```python
from build123d import *

# Parameters (mm, degrees)
SKETCH1_R               = 1.75
SKETCH1_W               = 5
SKETCH1_H               = 20
SKETCH1_R_2             = 13
BOSS_EXTRUDE1_DEPTH     = 3
SKETCH3_R               = 7.5
SKETCH3_R_2             = 4.75
BOSS_EXTRUDE2_DEPTH     = 8
BOSS_EXTRUDE4_DEPTH     = 6
CUT_EXTRUDE3_DEPTH      = 21
CUT_EXTRUDE3_DEPTH_BACK = 10
SKETCH1_5_R             = 1.75
CUT_EXTRUDE4_REACH      = 163.251
SKETCH10_R              = 6
CUT_EXTRUDE5_REACH      = 163.251
SKETCH11_R              = 6


with BuildPart() as part:
    # Sketch1 → Boss-Extrude1 (new body)
    with BuildSketch(Plane.XY):
        with BuildLine():
            Line((45.254833996, 60.811183182), (24.04163056, 39.597979746))
            Line((24.04163056, 39.597979746), (19.192388155, 34.748737342))
            ThreePointArc((19.192388155, 34.748737342), (15.948154667, 32.581009828), (12.121320344, 31.819805153))
            Line((12.121320344, 31.819805153), (-12.121320344, 31.819805153))
            ThreePointArc((-12.121320344, 31.819805153), (-15.948154667, 32.581009828), (-19.192388155, 34.748737342))
            Line((-19.192388155, 34.748737342), (-24.04163056, 39.597979746))
            Line((-24.04163056, 39.597979746), (-45.254833996, 60.811183182))
            Line((-45.254833996, 60.811183182), (-60.811183182, 45.254833996))
            Line((-60.811183182, 45.254833996), (-39.597979746, 24.04163056))
            Line((-39.597979746, 24.04163056), (-34.748737342, 19.192388155))
            ThreePointArc((-34.748737342, 19.192388155), (-32.581009828, 15.948154667), (-31.819805153, 12.121320344))
            Line((-31.819805153, 12.121320344), (-31.819805153, -12.121320344))
            ThreePointArc((-31.819805153, -12.121320344), (-32.581009828, -15.948154667), (-34.748737342, -19.192388155))
            Line((-34.748737342, -19.192388155), (-39.597979746, -24.04163056))
            Line((-39.597979746, -24.04163056), (-60.811183182, -45.254833996))
            Line((-60.811183182, -45.254833996), (-45.254833996, -60.811183182))
            Line((-45.254833996, -60.811183182), (-24.04163056, -39.597979746))
            Line((-24.04163056, -39.597979746), (-19.192388155, -34.748737342))
            ThreePointArc((-19.192388155, -34.748737342), (-15.948154667, -32.581009828), (-12.121320344, -31.819805153))
            Line((-12.121320344, -31.819805153), (12.121320344, -31.819805153))
            ThreePointArc((12.121320344, -31.819805153), (15.948154667, -32.581009828), (19.192388155, -34.748737342))
            Line((19.192388155, -34.748737342), (24.04163056, -39.597979746))
            Line((24.04163056, -39.597979746), (45.254833996, -60.811183182))
            Line((45.254833996, -60.811183182), (60.811183182, -45.254833996))
            Line((60.811183182, -45.254833996), (39.597979746, -24.04163056))
            Line((39.597979746, -24.04163056), (34.748737342, -19.192388155))
            ThreePointArc((34.748737342, -19.192388155), (32.581009828, -15.948154667), (31.819805153, -12.121320344))
            Line((31.819805153, -12.121320344), (31.819805153, 12.121320344))
            ThreePointArc((31.819805153, 12.121320344), (32.581009828, 15.948154667), (34.748737342, 19.192388155))
            Line((34.748737342, 19.192388155), (39.597979746, 24.04163056))
            Line((39.597979746, 24.04163056), (60.811183182, 45.254833996))
            Line((60.811183182, 45.254833996), (45.254833996, 60.811183182))
        make_face()
        with Locations((-40.305086528, -51.618795027)):
            Circle(SKETCH1_R, mode=Mode.SUBTRACT)
        with Locations((-51.618795027, -40.305086528)):
            Circle(SKETCH1_R, mode=Mode.SUBTRACT)
        with Locations((-26.162950904, -37.476659403)):
            Circle(SKETCH1_R, mode=Mode.SUBTRACT)
        with Locations((-37.476659403, -26.162950904)):
            Circle(SKETCH1_R, mode=Mode.SUBTRACT)
        with Locations((-15.25, -15.25)):
            Circle(SKETCH1_R, mode=Mode.SUBTRACT)
        with Locations((26.162950904, -37.476659403)):
            Circle(SKETCH1_R, mode=Mode.SUBTRACT)
        with Locations((40.305086528, -51.618795027)):
            Circle(SKETCH1_R, mode=Mode.SUBTRACT)
        with Locations((51.618795027, -40.305086528)):
            Circle(SKETCH1_R, mode=Mode.SUBTRACT)
        with Locations((15.25, -15.25)):
            Circle(SKETCH1_R, mode=Mode.SUBTRACT)
        with Locations((37.476659403, -26.162950904)):
            Circle(SKETCH1_R, mode=Mode.SUBTRACT)
        with Locations((-37.476659403, 26.162950904)):
            Circle(SKETCH1_R, mode=Mode.SUBTRACT)
        with Locations((-26.162950904, 0)):
            Rectangle(SKETCH1_W, SKETCH1_H, mode=Mode.SUBTRACT)
        with Locations((-15.25, 15.25)):
            Circle(SKETCH1_R, mode=Mode.SUBTRACT)
        with Locations((-51.618795027, 40.305086528)):
            Circle(SKETCH1_R, mode=Mode.SUBTRACT)
        with Locations((-40.305086528, 51.618795027)):
            Circle(SKETCH1_R, mode=Mode.SUBTRACT)
        with Locations((-26.162950904, 37.476659403)):
            Circle(SKETCH1_R, mode=Mode.SUBTRACT)
        Circle(SKETCH1_R_2, mode=Mode.SUBTRACT)
        with Locations((26.162950904, 0)):
            Rectangle(SKETCH1_W, SKETCH1_H, mode=Mode.SUBTRACT)
        with Locations((15.25, 15.25)):
            Circle(SKETCH1_R, mode=Mode.SUBTRACT)
        with Locations((37.476659403, 26.162950904)):
            Circle(SKETCH1_R, mode=Mode.SUBTRACT)
        with Locations((26.162950904, 37.476659403)):
            Circle(SKETCH1_R, mode=Mode.SUBTRACT)
        with Locations((51.618795027, 40.305086528)):
            Circle(SKETCH1_R, mode=Mode.SUBTRACT)
        with Locations((40.305086528, 51.618795027)):
            Circle(SKETCH1_R, mode=Mode.SUBTRACT)
    extrude(amount=BOSS_EXTRUDE1_DEPTH)

    # Sketch3 → Boss-Extrude2 (add)
    # profile 1 of 4: a face of its own
    with BuildSketch(Plane.XY):
        with Locations((-40.001785669, 40.001785669)):
            Circle(SKETCH3_R)
        with Locations((-40.001785669, 40.001785669)):
            Circle(SKETCH3_R_2, mode=Mode.SUBTRACT)
    # profile 2 of 4: a face of its own
    with BuildSketch(Plane.XY):
        with Locations(Location((-40.001785669, -40.001785669, 0), (0, 0, 180))):
            Circle(SKETCH3_R)
        with Locations((-40.001785669, -40.001785669)):
            Circle(SKETCH3_R_2, mode=Mode.SUBTRACT)
    # profile 3 of 4: a face of its own
    with BuildSketch(Plane.XY):
        with Locations((40.001785669, -40.001785669)):
            Circle(SKETCH3_R)
        with Locations((40.001785669, -40.001785669)):
            Circle(SKETCH3_R_2, mode=Mode.SUBTRACT)
    # profile 4 of 4: a face of its own
    with BuildSketch(Plane.XY):
        with Locations(Location((40.001785669, 40.001785669, 0), (0, 0, 180))):
            Circle(SKETCH3_R)
        with Locations((40.001785669, 40.001785669)):
            Circle(SKETCH3_R_2, mode=Mode.SUBTRACT)
    extrude(amount=-BOSS_EXTRUDE2_DEPTH)

    # Sketch7 → Boss-Extrude4 (add)
    with BuildSketch(Plane.XY.offset(3)):
        Polygon((-34.748737342, 19.192388155), (-19.192388155, 34.748737342), (-45.254833996, 60.811183182), (-60.811183182, 45.254833996), align=None)
        Polygon((-60.811183182, -45.254833996), (-34.748737342, -19.192388155), (-19.192388155, -34.748737342), (-45.254833996, -60.811183182), align=None)
        Polygon((34.748737342, -19.192388155), (19.192388155, -34.748737342), (45.254833996, -60.811183182), (60.811183182, -45.254833996), align=None)
        Polygon((60.811183182, 45.254833996), (34.748737342, 19.192388155), (19.192388155, 34.748737342), (45.254833996, 60.811183182), align=None)
    extrude(amount=BOSS_EXTRUDE4_DEPTH)

    # Sketch1<5> → Cut-Extrude3 (cut, two sides: drawn at the far end of the back side and taken through both)
    with BuildSketch(Plane.XY.offset(-CUT_EXTRUDE3_DEPTH_BACK)):
        with Locations(Location((-37.476659403, -26.162950904, 0), (0, 0, 180))):
            Circle(SKETCH1_5_R)
        with Locations(Location((-26.162950904, -37.476659403, 0), (0, 0, 180))):
            Circle(SKETCH1_5_R)
        with Locations(Location((-40.305086528, -51.618795027, 0), (0, 0, 180))):
            Circle(SKETCH1_5_R)
        with Locations(Location((-51.618795027, -40.305086528, 0), (0, 0, 180))):
            Circle(SKETCH1_5_R)
        with Locations(Location((26.162950904, 37.476659403, 0), (0, 0, 180))):
            Circle(SKETCH1_5_R)
        with Locations(Location((37.476659403, 26.162950904, 0), (0, 0, 180))):
            Circle(SKETCH1_5_R)
        with Locations(Location((51.618795027, 40.305086528, 0), (0, 0, 180))):
            Circle(SKETCH1_5_R)
        with Locations(Location((40.305086528, 51.618795027, 0), (0, 0, 180))):
            Circle(SKETCH1_5_R)
        with Locations((40.305086528, -51.618795027)):
            Circle(SKETCH1_5_R)
        with Locations((51.618795027, -40.305086528)):
            Circle(SKETCH1_5_R)
        with Locations((37.476659403, -26.162950904)):
            Circle(SKETCH1_5_R)
        with Locations((26.162950904, -37.476659403)):
            Circle(SKETCH1_5_R)
        with Locations((-51.618795027, 40.305086528)):
            Circle(SKETCH1_5_R)
        with Locations((-40.305086528, 51.618795027)):
            Circle(SKETCH1_5_R)
        with Locations((-26.162950904, 37.476659403)):
            Circle(SKETCH1_5_R)
        with Locations((-37.476659403, 26.162950904)):
            Circle(SKETCH1_5_R)
    extrude(amount=CUT_EXTRUDE3_DEPTH + CUT_EXTRUDE3_DEPTH_BACK, mode=Mode.SUBTRACT)

    # Cut-Extrude4: up to this face of the body (flat: up to its plane)
    cut_extrude4_end = Plane(part.part.faces().sort_by_distance((53.033008589, -53.033008589, 4.5))[0])
    # Sketch10 → Cut-Extrude4 (cut, up to the picked face)
    with BuildSketch(Plane(origin=(-53.033008589, 53.033008589, 0), x_dir=(0, 0, 1), z_dir=(-0.7071067811865477, 0.7071067811865474, 0)), mode=Mode.PRIVATE) as cut_extrude4_sk1:
        with Locations((11.5, 0)):
            Circle(SKETCH10_R)
    cut_extrude4_tool1 = split(extrude(cut_extrude4_sk1.sketch, amount=-CUT_EXTRUDE4_REACH, mode=Mode.PRIVATE), bisect_by=cut_extrude4_end, keep=Keep.BOTH, mode=Mode.PRIVATE)
    add(cut_extrude4_tool1.solids().sort_by(Axis((-53.033009, 53.033009, 11.5), (0.7071067811865477, -0.7071067811865474, 0)))[0], mode=Mode.SUBTRACT)

    # Cut-Extrude5: up to this face of the body (flat: up to its plane)
    cut_extrude5_end = Plane(part.part.faces().sort_by_distance((-53.033008589, -53.033008589, 4.5))[0])
    # Sketch11 → Cut-Extrude5 (cut, up to the picked face)
    with BuildSketch(Plane(origin=(53.033008589, 53.033008589, 0), x_dir=(0.7071067811865552, -0.7071067811865398, 0), z_dir=(0.7071067811865398, 0.7071067811865552, 0)), mode=Mode.PRIVATE) as cut_extrude5_sk1:
        with Locations((0, -11.5)):
            Circle(SKETCH11_R)
    cut_extrude5_tool1 = split(extrude(cut_extrude5_sk1.sketch, amount=-CUT_EXTRUDE5_REACH, mode=Mode.PRIVATE), bisect_by=cut_extrude5_end, keep=Keep.BOTH, mode=Mode.PRIVATE)
    add(cut_extrude5_tool1.solids().sort_by(Axis((53.033009, 53.033009, 11.5), (-0.7071067811865398, -0.7071067811865552, 0)))[0], mode=Mode.SUBTRACT)


solid = part.part
```
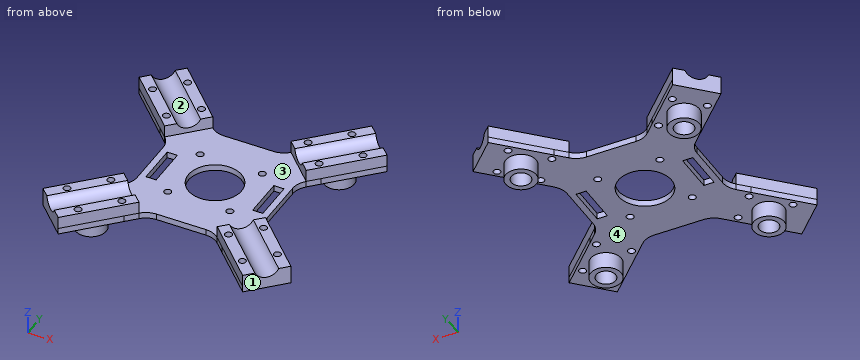
Could you check a few things on this model? Use its own coordinates, in mm. Face numbers are marked on the shaded views. A direction names the side the tool comes from. Round coordinates to 2 decimals unless told otherwise and drop trailing zeros. Order: outer loops, then holes, each group sorted by start corner. A loop starts at its lowest first (then second) coordinate and runs counter-clockwise, first axis right, second up. Notation, with made-up numbers: M -31,12.25 L -2,12.25 A25 cw -2,44.25 Z; hole C 81.25,24.25 d4. An arc over 180 degrees is marked long. One line per question, with ' | ' between items. Start each with the question number.
(1) Suppose I cut it at B-B on y = 0. List the corners of the cut face in (x, z) for me.
(2) Please list where these lines run through material, in increasing order: line 1 along X through (y, z) = (52.5, 2.25); line 2 along X through (y, z) = (-38, -4.5); line 3 along Z through (x, y) = (17, -14).
(3) Suppose I cut it at C-C on z = -4. List the corners of the cut face in (x, y) for me.
(4) For P1, Ø3, axis at x = -42, y = -39.5, coming from the -Z side; P2, Ø6, axis at y = 41, z = 2.5, coming from the -X side; P3, Ø8, axis at x = -10.5, y = 17, coming from the +Z side, each with a flat end and sliding along its axis, tell me the tip position at first contact or that it passes through.
(5) Thinking about a two-plate mould opening in Y: for the marked faces 1 and 2, which applies, +Y half, -Y half, draft (parallel to the pull), parting line (faces both ways), or undercut?
(6) For the marked faces 3 and 4, which set-ups out of +Z, -Z, +X, -X, +Y, -Y let a thin tool reach every point of the face, with its end or its side?
(7) Suppose I cut it at D-D on z = 7. Count the separate pieces of the cut face and the enclosed holes in it, then the cut area to 3 significant figures.
(8) Suppose I cut it at A-A on x = 0. List the corners of the cut face in (y, z) for me, then the cut area to 3 significant figures.
Geometry results:
1) outline: M -31.82,0 L -28.66,0 L -28.66,3 L -31.82,3 Z; M -23.66,0 L -13,0 L -13,3 L -23.66,3 Z; M 13,0 L 23.66,0 L 23.66,3 L 13,3 Z; M 28.66,0 L 31.82,0 L 31.82,3 L 28.66,3 Z
2) line 1: -53.57 to -41.82, -38.79 to -36.94, 36.94 to 38.79, 41.82 to 53.57 | line 2: -47.23 to -44.31, -35.69 to -32.77, 32.77 to 35.69, 44.31 to 47.23 | line 3: 0 to 3
3) outline: C -40,-40 d15; C -40,40 d15; C 40,-40 d15; C 40,40 d15; hole C -40,-40 d9.5; hole C -40,40 d9.5; hole C 40,-40 d9.5; hole C 40,40 d9.5
4) P1: z = 0 | P2: x = -59.56 | P3: z = 3
5) face 1: -Y half | face 2: undercut
6) face 3: +Z | face 4: -Z
7) separate pieces: 8 | enclosed holes: 16 | area: 1,920 mm²
8) outline: M -31.82,0 L -13,0 L -13,3 L -31.82,3 Z; M 13,0 L 31.82,0 L 31.82,3 L 13,3 Z | area: 113 mm²
